from build123d import *

# Parameters (mm, degrees)
SKETCH_W     = 587.5
SKETCH_H     = 340
PAD_DEPTH    = 10
SKETCH001_W  = 587.5
SKETCH001_H  = 45
PAD001_DEPTH = 60
SKETCH002_W  = 587.5
SKETCH002_H  = 45
PAD002_DEPTH = 60
SKETCH003_W  = 45
SKETCH003_H  = 250
PAD003_DEPTH = 60
SKETCH004_W  = 45
SKETCH004_H  = 250
PAD004_DEPTH = 60
SKETCH005_W  = 497.5
SKETCH005_H  = 30
PAD005_DEPTH = 60


with BuildPart() as part:
    # Sketch → Pad (new body)
    with BuildSketch(Plane.XY):
        with Locations((278.206882, -276.545756)):
            Rectangle(SKETCH_W, SKETCH_H)
    extrude(amount=PAD_DEPTH)

    # Sketch001 (on Face6 of Pad) → Pad001 (join)
    with BuildSketch(Plane.XY.offset(10)):
        with Locations((278.206882, -129.045756)):
            Rectangle(SKETCH001_W, SKETCH001_H)
    extrude(amount=PAD001_DEPTH)

    # Sketch002 (on Face3 of Pad001) → Pad002 (join)
    with BuildSketch(Plane.XY.offset(10)):
        with Locations((278.206882, -424.045756)):
            Rectangle(SKETCH002_W, SKETCH002_H)
    extrude(amount=PAD002_DEPTH)

    # Sketch003 (on Face3 of Pad002) → Pad003 (join)
    with BuildSketch(Plane.XY.offset(10)):
        with Locations((6.956882, -276.545756)):
            Rectangle(SKETCH003_W, SKETCH003_H)
    extrude(amount=PAD003_DEPTH)

    # Sketch004 (on Face6 of Pad003) → Pad004 (join)
    with BuildSketch(Plane.XY.offset(10)):
        with Locations((549.456882, -276.545756)):
            Rectangle(SKETCH004_W, SKETCH004_H)
    extrude(amount=PAD004_DEPTH)

    # Sketch005 (on Face11 of Pad004) → Pad005 (join)
    with BuildSketch(Plane.XY.offset(10)):
        with Locations((278.206882, -276.545756)):
            Rectangle(SKETCH005_W, SKETCH005_H)
    extrude(amount=PAD005_DEPTH)


solid = part.part
Build history of the part. All positions in model axes, mm. A direction names the side the tool comes from. Round coordinates to 2 decimals unless told otherwise and drop trailing zeros. Loops run counter-clockwise (first coordinate to the right, second up) from the corner with the lowest first, then second, coordinate; pieces in that order, holes last. Notation, with made-up numbers: (59.5, -19) -> (115.5, -19) arc R27 ccw to (115.5, 7) -> close; hole circle Ø3 at (72.5, 44). An arc over 180 degrees is marked (long way). Answer in a Markdown table with one row per item.
Item 1: Drill centre lines: L1, parallel to Y at x = 224.5, z = 49; L2, parallel to X at y = -306.5, z = 37; L3, parallel to Z at x = 211, y = -391. Where is each one in solid material? Low to high. Write a range as [from, to].
Answers below:
| item | result |
|---|---|
| L1 | y = [-446.55, -401.55], [-291.55, -261.55], [-151.55, -106.55] |
| L2 | x = [-15.54, 29.46], [526.96, 571.96] |
| L3 | z = [0, 10] |
Item 2: Saw through at A-A (z = 54). Write the cut outline in (x, y).
Answers below:
| item | result |
|---|---|
| outline | (-15.54, -446.55) -> (571.96, -446.55) -> (571.96, -106.55) -> (-15.54, -106.55) -> close; hole (29.46, -401.55) -> (526.96, -401.55) -> (526.96, -291.55) -> (29.46, -291.55) -> close; hole (29.46, -261.55) -> (526.96, -261.55) -> (526.96, -151.55) -> (29.46, -151.55) -> close |
Item 3: Which spindle directions (+Z, -Z, +X, -X, +Y, -Y) get a long thin tool onto all of the face, cutting with end or side? Do faces 4 (the flat face through (274, -274, 0)), 5 (the flat face through (526.957, -207, 40)). Say none if no direction does.
Answers below:
| item | result |
|---|---|
| face 4 | -Z, +X, -X, +Y, -Y |
| face 5 | +Z |
Item 4: Saw through at B-B (y = -379). Write the cut outline in (x, z).
Answers below:
| item | result |
|---|---|
| outline | (-15.54, 0) -> (571.96, 0) -> (571.96, 70) -> (526.96, 70) -> (526.96, 10) -> (29.46, 10) -> (29.46, 70) -> (-15.54, 70) -> close |
Item 5: Mould opens along X. For faces 1 (the flat face through (-15.543, -279, 35)), 2 (the flat face through (274, -274, 70)), 3 (the flat face through (275, -346, 10)) say: +X half, -X half, draft (parallel to the pull), parting line (faces both ways), or undercut.
Answers below:
| item | result |
|---|---|
| face 1 | -X half |
| face 2 | draft |
| face 3 | undercut |
Item 6: Saw through at C-C (x = 105.5). Write the cut outline in (y, z), and give its area (3 significant figures).
Answers below:
| item | result |
|---|---|
| outline | (-446.55, 0) -> (-106.55, 0) -> (-106.55, 70) -> (-151.55, 70) -> (-151.55, 10) -> (-261.55, 10) -> (-261.55, 70) -> (-291.55, 70) -> (-291.55, 10) -> (-401.55, 10) -> (-401.55, 70) -> (-446.55, 70) -> close |
| area | 10,600 mm² |
Item 7: Pin check, flat tip, straight feed: pin 1 (6 mm diameter, centred on x = 163, y = -334.5, fed in from +Z). Stop position of the tip, or through.
Answers below:
| item | result |
|---|---|
| pin 1 | stops at z = 10 |
